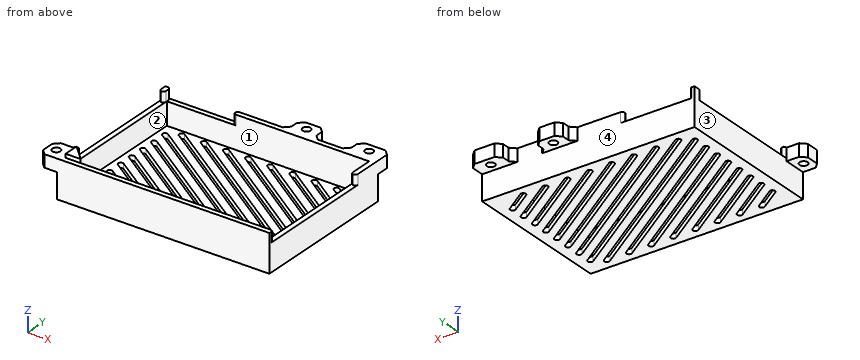
from build123d import *

# Parameters (mm, degrees)
SKETCH_1_W          = 84.5
SKETCH_1_H          = 59.5
EXTRUDE_1_DEPTH     = 2
SKETCH_2_W          = 84.5
SKETCH_2_H          = 59.5
SKETCH_2_W_2        = 80.5
SKETCH_2_H_2        = 55.5
EXTRUDE_2_DEPTH     = 13
SKETCH_3_W          = 26.5
SKETCH_3_H          = 4
CUT_EXTRUDE_1_DEPTH = 2
SKETCH_4_W          = 4
SKETCH_4_H          = 46
CUT_EXTRUDE_2_DEPTH = 2
SKETCH_5_W          = 4
SKETCH_5_H          = 45.5
CUT_EXTRUDE_3_DEPTH = 2
CUT_EXTRUDE_4_DEPTH = 105.160933176
SKETCH_9_W          = 7
SKETCH_9_H          = 9
SKETCH_9_R          = 1.6
EXTRUDE_5_DEPTH     = 5
FILLET_1_R          = 1
EXTRUDE_8_DEPTH     = 3
CHAMFER_4_SIZE      = 2
SKETCH_16_W         = 12
SKETCH_16_H         = 7
SKETCH_16_R         = 1.6
SKETCH_16_W_2       = 10
EXTRUDE_9_DEPTH     = 5
CHAMFER_5_SIZE      = 2


with BuildPart() as part:
    # 草图1 → 凸台-拉伸1 (new body)
    with BuildSketch(Plane.XY):
        with Locations((42.25, 29.75)):
            Rectangle(SKETCH_1_W, SKETCH_1_H)
    extrude(amount=EXTRUDE_1_DEPTH)

    # 草图2 → 凸台-拉伸2 (add)
    with BuildSketch(Plane.XY.offset(2)):
        with Locations((42.25, 29.75)):
            Rectangle(SKETCH_2_W, SKETCH_2_H)
        with Locations((42.25, 29.75)):
            Rectangle(SKETCH_2_W_2, SKETCH_2_H_2, mode=Mode.SUBTRACT)
    extrude(amount=EXTRUDE_2_DEPTH)

    # 草图3 → 切除-拉伸1 (cut)
    with BuildSketch(Plane(origin=(0, 59.5, 0), x_dir=(1, 0, 0), z_dir=(0, 1, 0))):
        with Locations((15.25, -13)):
            Rectangle(SKETCH_3_W, SKETCH_3_H)
    extrude(amount=-CUT_EXTRUDE_1_DEPTH, mode=Mode.SUBTRACT)

    # 草图4 → 切除-拉伸2 (cut)
    with BuildSketch(Plane.ZY):
        with Locations((13, 33)):
            Rectangle(SKETCH_4_W, SKETCH_4_H)
    extrude(amount=-CUT_EXTRUDE_2_DEPTH, mode=Mode.SUBTRACT)

    # 草图5 → 切除-拉伸3 (cut)
    with BuildSketch(Plane(origin=(84.5, 0, 0), x_dir=(0, 0, -1), z_dir=(1, 0, 0))):
        with Locations((-13, 24.75)):
            Rectangle(SKETCH_5_W, SKETCH_5_H)
    extrude(amount=-CUT_EXTRUDE_3_DEPTH, mode=Mode.SUBTRACT)

    # 草图6 → 切除-拉伸4 (cut, through all)
    with BuildSketch(Plane.XY.offset(2)):
        with BuildLine():
            Line((5.567613453, 16.779459118), (22.810337711, 4.89161817))
            ThreePointArc((22.810337711, 4.89161817), (23.066019447, 3.500709528), (21.675110805, 3.245027793))
            Line((21.675110805, 3.245027793), (4.432386547, 15.132868741))
            ThreePointArc((4.432386547, 15.132868741), (4.176704811, 16.523777383), (5.567613453, 16.779459118))
        make_face()
        with BuildLine():
            Line((5.567613453, 22.852614978), (31.619149364, 4.89161817))
            ThreePointArc((31.619149364, 4.89161817), (31.8748311, 3.500709528), (30.483922458, 3.245027793))
            Line((30.483922458, 3.245027793), (4.432386547, 21.206024601))
            ThreePointArc((4.432386547, 21.206024601), (4.176704811, 22.596933243), (5.567613453, 22.852614978))
        make_face()
        with BuildLine():
            Line((5.567613453, 28.925770838), (40.427961017, 4.89161817))
            ThreePointArc((40.427961017, 4.89161817), (40.683642752, 3.500709528), (39.29273411, 3.245027793))
            Line((39.29273411, 3.245027793), (4.432386547, 27.279180461))
            ThreePointArc((4.432386547, 27.279180461), (4.176704811, 28.670089102), (5.567613453, 28.925770838))
        make_face()
        with BuildLine():
            Line((5.567613453, 34.998926698), (49.236772669, 4.89161817))
            ThreePointArc((49.236772669, 4.89161817), (49.492454405, 3.500709528), (48.101545763, 3.245027793))
            Line((48.101545763, 3.245027793), (4.432386547, 33.35233632))
            ThreePointArc((4.432386547, 33.35233632), (4.176704811, 34.743244962), (5.567613453, 34.998926698))
        make_face()
        with BuildLine():
            Line((5.567613453, 41.072082558), (58.045584322, 4.89161817))
            ThreePointArc((58.045584322, 4.89161817), (58.301266057, 3.500709528), (56.910357415, 3.245027793))
            Line((56.910357415, 3.245027793), (4.432386547, 39.42549218))
            ThreePointArc((4.432386547, 39.42549218), (4.176704811, 40.816400822), (5.567613453, 41.072082558))
        make_face()
        with BuildLine():
            Line((5.567613453, 47.145238418), (66.854395974, 4.89161817))
            ThreePointArc((66.854395974, 4.89161817), (67.11007771, 3.500709528), (65.719169068, 3.245027793))
            Line((65.719169068, 3.245027793), (4.432386547, 45.49864804))
            ThreePointArc((4.432386547, 45.49864804), (4.176704811, 46.889556682), (5.567613453, 47.145238418))
        make_face()
        with BuildLine():
            Line((9.972019279, 56.254972207), (80.067613453, 7.9281961))
            ThreePointArc((80.067613453, 7.9281961), (80.323295189, 6.537287458), (78.932386547, 6.281605723))
            Line((78.932386547, 6.281605723), (8.836792373, 54.60838183))
            ThreePointArc((8.836792373, 54.60838183), (8.581110638, 55.999290472), (9.972019279, 56.254972207))
        make_face()
        with BuildLine():
            Line((5.567613453, 53.218394277), (75.663207627, 4.89161817))
            ThreePointArc((75.663207627, 4.89161817), (75.918889362, 3.500709528), (74.527980721, 3.245027793))
            Line((74.527980721, 3.245027793), (4.432386547, 51.5718039))
            ThreePointArc((4.432386547, 51.5718039), (4.176704811, 52.962712542), (5.567613453, 53.218394277))
        make_face()
        with BuildLine():
            Line((5.567613453, 10.706303259), (14.001526059, 4.89161817))
            ThreePointArc((14.001526059, 4.89161817), (14.257207795, 3.500709528), (12.866299153, 3.245027793))
            Line((12.866299153, 3.245027793), (4.432386547, 9.059712881))
            ThreePointArc((4.432386547, 9.059712881), (4.176704811, 10.450621523), (5.567613453, 10.706303259))
        make_face()
        with BuildLine():
            Line((18.780830932, 56.254972207), (80.067613453, 14.00135196))
            ThreePointArc((80.067613453, 14.00135196), (80.323295189, 12.610443318), (78.932386547, 12.354761582))
            Line((78.932386547, 12.354761582), (17.645604026, 54.60838183))
            ThreePointArc((17.645604026, 54.60838183), (17.38992229, 55.999290472), (18.780830932, 56.254972207))
        make_face()
        with BuildLine():
            Line((27.589642585, 56.254972207), (80.067613453, 20.07450782))
            ThreePointArc((80.067613453, 20.07450782), (80.323295189, 18.683599178), (78.932386547, 18.427917442))
            Line((78.932386547, 18.427917442), (26.454415678, 54.60838183))
            ThreePointArc((26.454415678, 54.60838183), (26.198733943, 55.999290472), (27.589642585, 56.254972207))
        make_face()
        with BuildLine():
            Line((36.398454237, 56.254972207), (80.067613453, 26.14766368))
            ThreePointArc((80.067613453, 26.14766368), (80.323295189, 24.756755038), (78.932386547, 24.501073302))
            Line((78.932386547, 24.501073302), (35.263227331, 54.60838183))
            ThreePointArc((35.263227331, 54.60838183), (35.007545595, 55.999290472), (36.398454237, 56.254972207))
        make_face()
        with BuildLine():
            Line((45.20726589, 56.254972207), (80.067613453, 32.220819539))
            ThreePointArc((80.067613453, 32.220819539), (80.323295189, 30.829910898), (78.932386547, 30.574229162))
            Line((78.932386547, 30.574229162), (44.072038983, 54.60838183))
            ThreePointArc((44.072038983, 54.60838183), (43.816357248, 55.999290472), (45.20726589, 56.254972207))
        make_face()
        with BuildLine():
            Line((54.016077542, 56.254972207), (80.067613453, 38.293975399))
            ThreePointArc((80.067613453, 38.293975399), (80.323295189, 36.903066757), (78.932386547, 36.647385022))
            Line((78.932386547, 36.647385022), (52.880850636, 54.60838183))
            ThreePointArc((52.880850636, 54.60838183), (52.6251689, 55.999290472), (54.016077542, 56.254972207))
        make_face()
        with BuildLine():
            Line((62.824889195, 56.254972207), (80.067613453, 44.367131259))
            ThreePointArc((80.067613453, 44.367131259), (80.323295189, 42.976222617), (78.932386547, 42.720540882))
            Line((78.932386547, 42.720540882), (61.689662289, 54.60838183))
            ThreePointArc((61.689662289, 54.60838183), (61.433980553, 55.999290472), (62.824889195, 56.254972207))
        make_face()
        with BuildLine():
            Line((71.633700847, 56.254972207), (80.067613453, 50.440287119))
            ThreePointArc((80.067613453, 50.440287119), (80.323295189, 49.049378477), (78.932386547, 48.793696741))
            Line((78.932386547, 48.793696741), (70.498473941, 54.60838183))
            ThreePointArc((70.498473941, 54.60838183), (70.242792205, 55.999290472), (71.633700847, 56.254972207))
        make_face()
    extrude(amount=-CUT_EXTRUDE_4_DEPTH, mode=Mode.SUBTRACT)

    # 草图9 → 凸台-拉伸5 (add)
    with BuildSketch(Plane.XY.offset(15)):
        with Locations((-3.5, 4.5)):
            Rectangle(SKETCH_9_W, SKETCH_9_H)
        with Locations((-3.5, 4.5)):
            Circle(SKETCH_9_R, mode=Mode.SUBTRACT)
    extrude(amount=-EXTRUDE_5_DEPTH)

    # 圆角1
    fillet_1_edges = [part.edges().sort_by_distance(p)[0] for p in [
        (2, 10, 13),
        (84.5, 47.5, 13),
        (82.5, 47.5, 13),
        (84.5, 2, 13),
        (28.5, 57.5, 13),
        (28.5, 59.5, 13),
        (2, 59.5, 13),
        (2, 56, 13),
        (0, 56, 13),
        (0, 10, 13),
    ]]
    fillet(fillet_1_edges, radius=FILLET_1_R - 0.0001)  # a hair under: the kernel refuses the full size

    # 草图15 → 凸台-拉伸8 (add)
    with BuildSketch(Plane.XY.offset(16.5)):
        Polygon((2, 2), (2, 8), (8, 2), align=None)
    extrude(amount=-EXTRUDE_8_DEPTH)

    # 倒角4
    chamfer_4_edges = [part.edges().sort_by_distance(p)[0] for p in [
        (5, 2, 13.5),
        (2, 5, 13.5),
    ]]
    chamfer(chamfer_4_edges, length=CHAMFER_4_SIZE)

    # 草图16 → 凸台-拉伸9 (add)
    # profile 1 of 2: a face of its own
    with BuildSketch(Plane.XY.offset(15)):
        with Locations((78.5, 63)):
            Rectangle(SKETCH_16_W, SKETCH_16_H)
        with Locations((78.5, 63)):
            Circle(SKETCH_16_R, mode=Mode.SUBTRACT)
    # profile 2 of 2: a face of its own
    with BuildSketch(Plane.XY.offset(15)):
        with Locations((53.62, 63)):
            Rectangle(SKETCH_16_W_2, SKETCH_16_H)
        with Locations((53.62, 63)):
            Circle(SKETCH_16_R, mode=Mode.SUBTRACT)
    extrude(amount=-EXTRUDE_9_DEPTH)

    # 倒角5
    chamfer_5_edges = [part.edges().sort_by_distance(p)[0] for p in [
        (-7, 0, 12.5),
        (-7, 9, 12.5),
        (84.5, 66.5, 12.5),
        (72.5, 59.5, 12.5),
        (72.5, 66.5, 12.5),
        (58.62, 66.5, 12.5),
        (58.62, 59.5, 12.5),
        (48.62, 59.5, 12.5),
        (48.62, 66.5, 12.5),
    ]]
    chamfer(chamfer_5_edges, length=CHAMFER_5_SIZE)


solid = part.part
Read the model definition and answer for the solid it produces. Units are mm, in the model's axes. Face numbers are marked on the shaded views. Coordinates: 2 decimals unless noted, no trailing zeros. Loops run counter-clockwise (first coordinate to the right, second up) from the corner with the lowest first, then second, coordinate; pieces in that order, holes last.
Q1. Consider probe 1 along Y at (x, z) = (66.5, 13.75); probe 2 along X at (y, z) = (44, 7); probe 3 along Y at (x, z) = (-3.5, 14). Determine where each line is inside the solid, lowest interval first.
Q2. The part is cut by section B-B on x = -3.5. Write down the section's boundary in (y, z), and give its area (3 significant figures).
Q3. The mould has two halves that part along Y. Classify the marked faces 1, 2, 3 and 4: +Y half, -Y half, draft (parallel to the pull), parting line (faces both ways), or undercut.
Q4. The part is cut by section C-C on z = 8. Write down the section's boundary in (x, y).
Q5. The part is cut by section A-A on y = 63. Write down the section's boundary in (x, z).
Q6. Each of these flat-tipped pins is pushed along its axis until it touches: pin 1 Ø2 at (y, z) = (38, 12.5) entering from -X; pin 2 Ø0.6 at (x, y) = (19, 59) entering from +Z; pin 3 Ø6 at (x, y) = (42.5, 52) entering from +Z; pin 4 Ø4 at (x, z) = (-1.5, 12.5) entering from +Y. Where does it stop, or does it pass through?
Results below:
1. probe 1: y = 0 to 2, 57.5 to 59.5
1. probe 2: x = 0 to 2, 82.5 to 84.5
1. probe 3: y = 0 to 2.9, 6.1 to 9
2. outline: (0, 10) - (2.9, 10) - (2.9, 15) - (0, 15) - close; (6.1, 10) - (9, 10) - (9, 15) - (6.1, 15) - close
2. area: 29.0 mm2
3. face 1: undercut
3. face 2: undercut
3. face 3: draft
3. face 4: +Y half
4. outline: (0, 0) - (84.5, 0) - (84.5, 59.5) - (0, 59.5) - close; hole (2, 2) - (82.5, 2) - (82.5, 57.5) - (2, 57.5) - close
5. outline: (48.62, 10) - (52.02, 10) - (52.02, 15) - (48.62, 15) - close; (55.22, 10) - (58.62, 10) - (58.62, 15) - (55.22, 15) - close; (72.5, 10) - (76.9, 10) - (76.9, 15) - (72.5, 15) - close; (80.1, 10) - (84.5, 10) - (84.5, 15) - (80.1, 15) - close
6. pin 1: passes through
6. pin 2: stops at z = 11
6. pin 3: stops at z = 2
6. pin 4: stops at y = 59.5
